Check sheet for the modelled part. Datum: model origin and axes. Units: mm. A direction names the side the tool comes from. Coordinates: 2 decimals unless noted, no trailing zeros. Loops run counter-clockwise (first coordinate to the right, second up) from the corner with the lowest first, then second, coordinate; pieces in that order, holes last.
Autodesk Inventor part; units mm, degrees
ref_plane "YZ Plane" through (0, 0, 0) normal (1, 0, 0) x (0, 1, 0)
ref_plane "XZ Plane" through (0, 0, 0) normal (0, 1, 0) x (-1, 0, 0)
ref_plane "XY Plane" through (0, 0, 0) normal (0, 0, 1) x (1, 0, 0)
sketch "Sketch1" plane through (0, 0, 0) normal (0, 0, 1) x (1, 0, 0)
  line L0 (0, 0) -> (0, 5)
  line L1 (0, 5) -> (110, 5)
  line L2 (110, 5) -> (110, 0)
  line L3 (110, 0) -> (0, 0)
  dimension "d0" = 110
  dimension "d1" = 10
revolve "Revolution1" add sketch "Sketch1" angle 360 about axis through (110, 0, 0) along (-1, 0, 0)
sketch "Sketch2" plane through (110, 0, 0) normal (1, 0, 0) x (0, 0, -1)
  circle A0 centre (0, 0) radius 5
hole "Hole1" at (110, 0, 0) direction (-1, 0, 0) diameter 4.134 depth 14.2
sketch "Sketch3" plane through (0, 0, 0) normal (-1, 0, 0) x (0, 0, 1)
  circle A0 centre (0, 0) radius 5
hole "Hole2" at (0, 0, 0) direction (1, 0, 0) diameter 4.134 depth 12
properties part number "1 part 21"
(1) Draft check along Z on faces 1 (the face through (0, 2, 1)), 2 (the face through (55.77, -1.08, -4.88)), 3 (the face through (6.08, 1.26, -1.64)). Enter one of: pulls with the +Z half, pulls with the -Z half, needs draft (parallel to the pull), parting line crosses it, or undercut.
(2) Section check D-D, the plane x = 37. Enter the section's corners in (y, z).
(3) Gauge pin test, flat ends, axial feed: P1, Ø1.5, axis at x = 74.5, z = 3, coming from the -Y side; P2, Ø4, axis at x = 91, y = 0.5, coming from the -Z side; P3, Ø1.5, axis at x = 73.5, z = 2.5, coming from the +Y side; P4, Ø5, axis at x = 45.5, z = -3, coming from the +Y side. Record the tip position at first contact, or that the pin passes through.
(4) Section check A-A, the plane x = 100. Enter the section's corners in (y, z).
(5) Section check B-B, the plane z = 0. Enter the section's corners in (x, y), plus the area to 3 significant figures.
(6) Set-up check for faces 4 (the face through (12, 0, 0)), 5 (the face through (95.8, 0, 0)), 6 (the face through (110, 2, 1)): record each of +Z, -Z, +X, -X, +Y, -Y from which the full face is reachable in a straight line by a thin tool's end or side.
(7) Scan lines: line 1 along Y through (x, z) = (99, 0); line 2 along X through (y, z) = (0, 0.75). Record each from-to range of solid material in increasing order.
Determined:
1. face 1: needs draft
1. face 2: parting line crosses it
1. face 3: undercut
2. outline: circle Ø10 at (0, 0)
3. P1: stops at y = -4.47
3. P2: stops at z = -5
3. P3: stops at y = 4.68
3. P4: stops at y = 4.97
4. outline: circle Ø10 at (0, 0); hole circle Ø4.13 at (0, 0)
5. outline: (0, -5) - (110, -5) - (110, -2.07) - (95.8, -2.07) - (95.8, 2.07) - (110, 2.07) - (110, 5) - (0, 5) - (0, 2.07) - (12, 2.07) - (12, -2.07) - (0, -2.07) - close
5. area: 992 mm2
6. face 4: -X
6. face 5: +X
6. face 6: +Z, -Z, +X, +Y, -Y
7. line 1: y = -5 to -2.07, 2.07 to 5
7. line 2: x = 12 to 95.8
